For this review, take the finished solid that the model builds, in its own axes (mm). Face numbers are marked on the shaded views. A direction names the side the tool comes from. Coordinates: 2 decimals unless noted, no trailing zeros. Write each loop counter-clockwise with the first axis right and the second up, starting at its lowest first coordinate (ties: lowest second). Pieces come first, ordered by that corner, then holes. Notation, with made-up numbers: (28, -0.5) -> (56, -0.5) arc R20 cw to (56, 20.5) -> close; hole circle Ø10 at (52.25, 82). An arc over 180 degrees is marked (long way). One line per item, written item: value. Start each with the question number.
1) Add section D-D (x = 4.5). State the section outline as (y, z) points, and give its area (3 significant figures).
2) Mouldability with a two-part tool opening along Z and no side actions: class the marked faces 3, 4 and 5 as released by +Z, released by -Z, zero draft, split by the parting line, or undercut.
3) Add section A-A (z = 0). State the section outline as (x, y) points, and give its area (3 significant figures).
4) Add section B-B (y = 0). State the section outline as (x, z) points.
5) For pin 1 Ø6 at (x, z) = (19, -1) entering from -Y; pin 2 Ø1.1 at (x, z) = (10.5, -24) entering from +Y; pin 3 Ø3 at (x, y) = (20, 9.5) entering from +Z; pin 4 Ø12 at (x, y) = (9.5, 7) entering from +Z, all flat-tipped, find the tip position at first contact; note any pin that passes through.
6) Machinability: for the marked faces 1 and 2, which of the approach directions +Z, -Z, +X, -X, +Y, -Y give a long, thin tool a straight path to every point of the face, cutting with its end or side? Answer none if there is none.
7) Add section C-C (x = 15.5). State the section outline as (y, z) points.
8) For probe 1 along Z at (x, y) = (10.33, 11.5); probe 2 along Z at (x, y) = (19.83, 18); probe 3 along X at (y, z) = (14, -16.5), list the stretches that pass through material, from the lowest coordinate up. Write a range as from..to.
from build123d import *

# Parameters (mm, degrees)
SKETCH1_R           = 31.6865
BOSS_EXTRUDE1_DEPTH = 26.9875
CUT_EXTRUDE1_DEPTH  = 20.32
SKETCH5_R           = 0.508
CUT_EXTRUDE2_DEPTH  = 12.7
SKETCH6_R           = 0.508
CUT_EXTRUDE3_DEPTH  = 3.556
SKETCH7_R           = 2.69875
BOSS_EXTRUDE2_DEPTH = 3.175
SKETCH11_R          = 2.69875
CUT_EXTRUDE6_DEPTH  = 3.175
SKETCH12_R          = 1.651
CUT_EXTRUDE7_DEPTH  = 9.017


with BuildPart() as part:
    # Sketch1 → Boss-Extrude1 (new body)
    with BuildSketch(Plane(origin=(0, 0, 0), x_dir=(0, 0, -1), z_dir=(1, 0, 0))):
        Circle(SKETCH1_R)
    extrude(amount=BOSS_EXTRUDE1_DEPTH)

    # Sketch3 → Cut-Extrude1 (cut)
    with BuildSketch(Plane(origin=(26.9875, 0, 0), x_dir=(0, 0, -1), z_dir=(1, 0, 0))):
        with BuildLine():
            Line((19.614864522, -8.95), (30.396246187, -8.95))
            ThreePointArc((30.396246187, -8.95), (30.911627748, -6.964592752), (31.297472458, -4.95))
            Line((31.297472458, -4.95), (19.614864522, -4.95))
            Line((19.614864522, -4.95), (19.614864522, 21.05))
            Line((19.614864522, 21.05), (23.683998443, 21.05))
            ThreePointArc((23.683998443, 21.05), (0, 31.6865), (-23.683998443, 21.05))
            Line((-23.683998443, 21.05), (-20.785135478, 21.05))
            Line((-20.785135478, 21.05), (-20.785135478, -10.95))
            Line((-20.785135478, -10.95), (19.614864522, -10.95))
            Line((19.614864522, -10.95), (19.614864522, -8.95))
        make_face()
    extrude(amount=-CUT_EXTRUDE1_DEPTH, mode=Mode.SUBTRACT)

    # Sketch5 → Cut-Extrude2 (cut)
    with BuildSketch(Plane(origin=(0, 21.05, 0), x_dir=(1, 0, 0), z_dir=(0, 1, 0))):
        with Locations((10.33, -24.932573059)):
            Circle(SKETCH5_R)
        with Locations((19.83, -24.932573059)):
            Circle(SKETCH5_R)
        with Locations((10.33, 23.762302103)):
            Circle(SKETCH5_R)
        with Locations((19.83, 23.762302103)):
            Circle(SKETCH5_R)
    extrude(amount=-CUT_EXTRUDE2_DEPTH, mode=Mode.SUBTRACT)

    # Sketch6 → Cut-Extrude3 (cut)
    with BuildSketch(Plane.ZY):
        with Locations((-1.539927539, 19.940627452)):
            Circle(SKETCH6_R)
    extrude(amount=-CUT_EXTRUDE3_DEPTH, mode=Mode.SUBTRACT)

    # Sketch7 → Boss-Extrude2 (add)
    with BuildSketch(Plane(origin=(6.6675, 0, 0), x_dir=(0, 0, -1), z_dir=(1, 0, 0))):
        Circle(SKETCH7_R)
    extrude(amount=-BOSS_EXTRUDE2_DEPTH)

    # Sketch11 → Cut-Extrude6 (cut)
    with BuildSketch(Plane(origin=(6.6675, 0, 0), x_dir=(0, 0, -1), z_dir=(1, 0, 0))):
        Circle(SKETCH11_R)
    extrude(amount=-CUT_EXTRUDE6_DEPTH, mode=Mode.SUBTRACT)

    # Sketch12 → Cut-Extrude7 (cut)
    with BuildSketch(Plane.ZY):
        Circle(SKETCH12_R)
    extrude(amount=-CUT_EXTRUDE7_DEPTH, mode=Mode.SUBTRACT)


solid = part.part
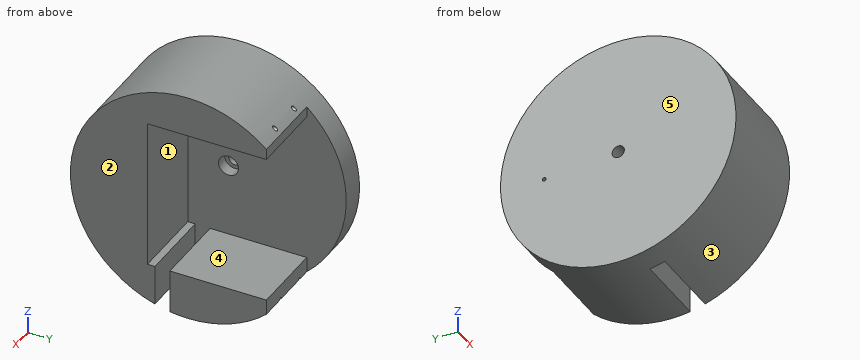
Numbers:
1. outline: circle Ø63.37 at (0, 0); hole circle Ø5.4 at (0, 0)
1. area: 3,130 mm²
2. face 3: split by the parting line
2. face 4: undercut
2. face 5: zero draft
3. outline: (0, -31.69) -> (26.99, -31.69) -> (26.99, -10.95) -> (6.67, -10.95) -> (6.67, -2.7) -> (3.49, -2.7) -> (3.49, -1.65) -> (0, -1.65) -> close; (0, 1.65) -> (3.49, 1.65) -> (3.49, 2.7) -> (6.67, 2.7) -> (6.67, 31.69) -> (0, 31.69) -> close
3. area: 815 mm²
4. outline: (0, -31.69) -> (26.99, -31.69) -> (26.99, -19.61) -> (6.67, -19.61) -> (6.67, -2.7) -> (3.49, -2.7) -> (3.49, -1.65) -> (0, -1.65) -> close; (0, 1.65) -> (3.49, 1.65) -> (3.49, 2.7) -> (6.67, 2.7) -> (6.67, 20.79) -> (26.99, 20.79) -> (26.99, 31.69) -> (0, 31.69) -> close
5. pin 1: y = -31.69
5. pin 2: y = 21.05
5. pin 3: z = 30.66
5. pin 4: z = 31.67
6. face 1: +X, +Y
6. face 2: +Z, -Z, +X, +Y, -Y
7. outline: (-10.95, -19.61) -> (-10.95, 20.79) -> (21.05, 20.79) -> (21.05, 23.68) arc R31.69 ccw (long way) to (-8.95, -30.4) -> (-8.95, -19.61) -> close; (-4.95, -31.3) arc R31.69 ccw to (21.05, -23.68) -> (21.05, -19.61) -> (-4.95, -19.61) -> close
8. probe 1: -29.53..-24.27, -23.25..-19.61, 20.79..24.42, 25.44..29.53
8. probe 2: -26.08..-24.27, -23.25..-19.61, 20.79..24.42, 25.44..26.08
8. probe 3: 0..6.67
